Check sheet for the drawn part. Datum: minimum x, y, z corner. Units: mm. Round coordinates to 2 decimals unless told otherwise and drop trailing zeros. Write each loop counter-clockwise with the first axis right and the second up, starting at its lowest first coordinate (ties: lowest second). Pieces come first, ordered by that corner, then holes. Notation, with made-up numbers: (-21, 83) -> (14, 83) arc R27 ccw to (14, 115) -> close; hole circle Ø3 at (-33.75, 8). An arc over 180 degrees is marked (long way). One line per item, written item: value. Start each with the question number.
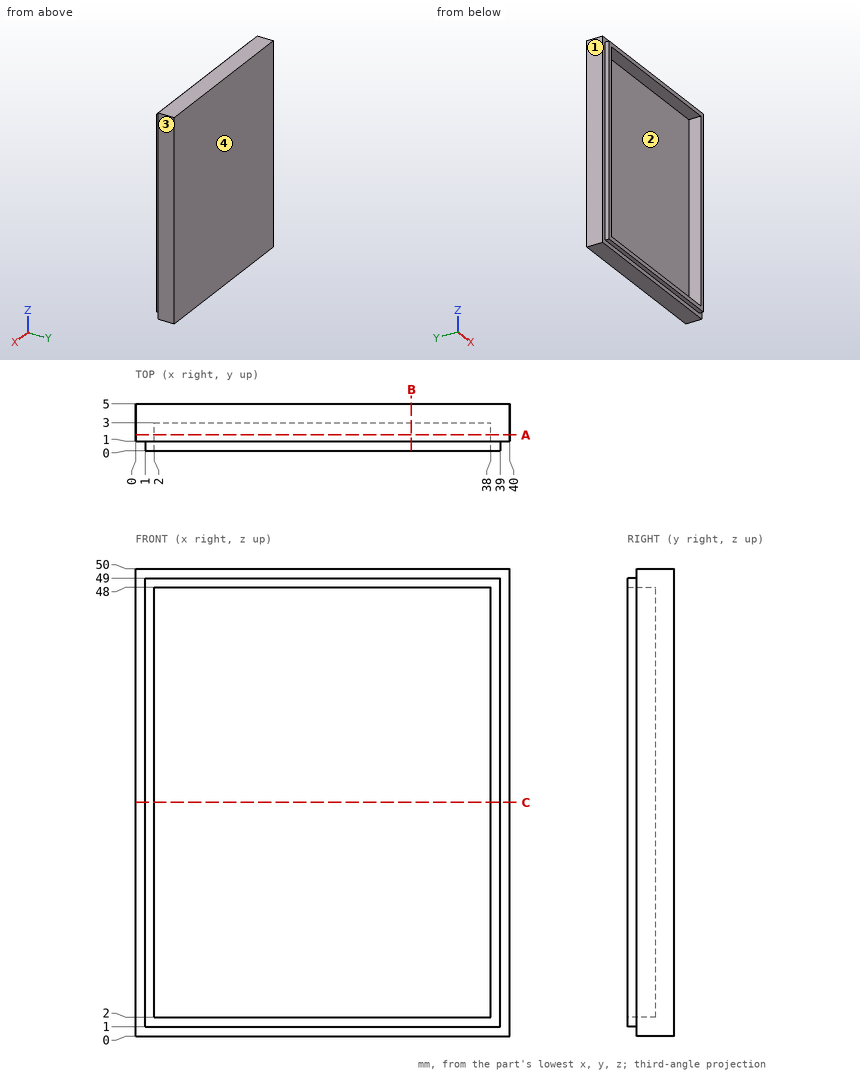
1. Cross-section at A-A (y = 1.7). Record the cut outline in (x, z).
2. Cross-section at B-B (x = 29.5). Record the cut outline in (y, z), plus the area to 3 significant figures.
3. Material ranges on probe 1 along Z at (x, y) = (26, 2.1); probe 2 along Z at (x, y) = (24, 0.6); probe 3 along X at (y, z) = (0.6, 41), recorded low to high.
4. Cross-section at C-C (z = 25). Record the cut outline in (x, y).
5. Release check for a two-part mould opening along X. For the marked faces 1, 2, 3 and 4 record: +X half, -X half, draft (parallel to the pull), parting line (faces both ways), or undercut.
6. Depth check by flat-ended pin: pin 1 Ø0.5 at (x, y) = (18, 0.5) entering from +Z; pin 2 Ø1.5 at (y, z) = (2, 28) entering from -X; pin 3 Ø0.5 at (y, z) = (0.5, 23) entering from +X; pin 4 Ø18 at (x, z) = (16, 21) entering from -Y. Enter the tip coordinate at first touch or a pass-through.
Working result:
1. outline: (0, 0) -> (40, 0) -> (40, 50) -> (0, 50) -> close; hole (2, 2) -> (38, 2) -> (38, 48) -> (2, 48) -> close
2. outline: (0, 1) -> (1, 1) -> (1, 0) -> (5, 0) -> (5, 50) -> (1, 50) -> (1, 49) -> (0, 49) -> (0, 48) -> (3, 48) -> (3, 2) -> (0, 2) -> close
2. area: 110 mm^2
3. probe 1: z = 0 to 2, 48 to 50
3. probe 2: z = 1 to 2, 48 to 49
3. probe 3: x = 1 to 2, 38 to 39
4. outline: (0, 1) -> (1, 1) -> (1, 0) -> (2, 0) -> (2, 3) -> (38, 3) -> (38, 0) -> (39, 0) -> (39, 1) -> (40, 1) -> (40, 5) -> (0, 5) -> close
5. face 1: -X half
5. face 2: undercut
5. face 3: +X half
5. face 4: draft
6. pin 1: stops at z = 49
6. pin 2: stops at x = 0
6. pin 3: stops at x = 39
6. pin 4: stops at y = 3
